from build123d import *

# Parameters (mm, degrees)
F1_DEPTH = 2.54
F2_R     = 11.6205
F3_DEPTH = 9.525
F4_SIZE  = 0.635
F5_R     = 3.175
F6_DEPTH = 2.541


with BuildPart() as f1:
    # F0 (on Top) → F1 (new body)
    with BuildSketch(Plane.XY):
        with BuildLine():
            Line((25.4, 4.7625), (8.951913, 10.724932))
            ThreePointArc((8.951913, 10.724932), (-13.97, 0), (8.951913, -10.724932))
            Line((8.951913, -10.724932), (25.4, -4.7625))
            ThreePointArc((25.4, -4.7625), (30.1625, 0), (25.4, 4.7625))
        make_face()
    extrude(amount=F1_DEPTH)

    # F2 (on face) → F3 (join)
    with BuildSketch(Plane.XY.offset(2.54)):
        with BuildLine():
            ThreePointArc((8.951913, -10.724932), (12.653441, -5.920417), (13.97, 0))
            ThreePointArc((13.97, 0), (12.653441, 5.920417), (8.951913, 10.724932))
            ThreePointArc((8.951913, 10.724932), (-13.97, 0), (8.951913, -10.724932))
        make_face()
        Circle(F2_R, mode=Mode.SUBTRACT)
    extrude(amount=F3_DEPTH)

    # F4
    f4_edges = [f1.edges().sort_by_distance(p)[0] for p in [
        (-11.6205, 0, 12.065),
    ]]
    chamfer(f4_edges, length=F4_SIZE)

    # F5 (on face) → F6 (cut, through all)
    with BuildSketch(Plane.XY.offset(2.54)):
        with Locations((25.4, 0)):
            Circle(F5_R)
    extrude(amount=-F6_DEPTH, mode=Mode.SUBTRACT)


solid = f1.part
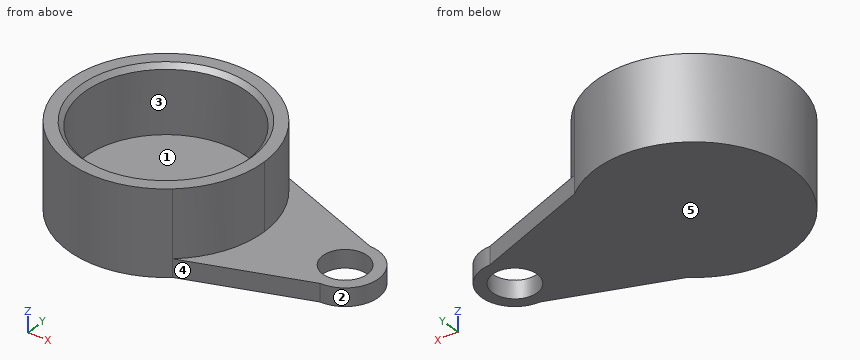
Source: CAD feature listing. Evaluate the final solid. Frame: model axes, mm. Face numbers are marked on the shaded views. A direction names the side the tool comes from. Give positions to 0.01 mm unless a question says otherwise; leave off trailing zeros. Write each loop counter-clockwise with the first axis right and the second up, starting at its lowest first coordinate (ties: lowest second). Pieces come first, ordered by that corner, then holes. Notation, with made-up numbers: M 37,34.5 L 89,34.5 A16 cw 89,58.5 Z; hole C -21,33 d4. An arc over 180 degrees is marked long. Return JSON: item names as keys, results as strings. Group by question number.
1) Material intervals for line 1 along X through (y, z) = (0.25, 9); line 2 along Y through (x, z) = (25.4, 0.6) (1 decimal); line 3 along Z through (x, y) = (1, -8.5), sorted ascending. Write a range as [from, to].
2) Cut plane C-C, the plane z = 7. Output: boundary loops of the cut face in (x, y), plus the area to 3 significant figures.
3) Pin query (flat end, axial travel): P1, Ø10.5, axis at x = 24.5, y = 3.5, coming from the +Z side; P2, Ø5, axis at y = 0.5, z = 8, coming from the +X side; P3, Ø4, axis at x = 12.5, z = 2.5, coming from the -Y side. Return the tip coordinate at first contact, or that it passes through.
4) Cut plane A-A, the plane x = 0. Output: boundary loops of the cut face in (y, z) (1 decimal), plus the area to 3 significant figures.
5) Set-up query: the marked faces 1 and 2. Return all of +Z, -Z, +X, -X, +Y, -Y with unobstructed straight access to the full face (end or side cutting, diameter ignored); none if empty.
6) Pull-direction query (Y, two-part tool) for the marked faces 3, 4 and 5; classes: pulls with the +Y half, pulls with the -Y half, needs draft (parallel to the pull), parting line crosses it, or undercut.
7) Cut plane D-D, the plane x = 15. Output: boundary loops of the cut face in (y, z), plus the area to 3 significant figures.
Recorded:
{
 "1": {"line 1": "x = [-13.97, -11.62], [11.62, 13.97]", "line 2": "y = [-4.8, -3.2], [3.2, 4.8]", "line 3": "z = [0, 2.54]"},
 "2": {"outline": "C 0,0 d27.94; hole C 0,0 d23.24", "area": "189 mm²"},
 "3": {"P1": "stops at z = 2.54", "P2": "stops at x = 13.97", "P3": "stops at y = -10.16"},
 "4": {"outline": "M -14,0 L 14,0 L 14,12.1 L 12.3,12.1 L 11.6,11.4 L 11.6,2.5 L -11.6,2.5 L -11.6,11.4 L -12.3,12.1 L -14,12.1 Z", "area": "115 mm²"},
 "5": {"face 1": "+Z", "face 2": "+Z, -Z, +X"},
 "6": {"face 3": "undercut", "face 4": "pulls with the -Y half", "face 5": "needs draft"},
 "7": {"outline": "M -8.53,0 L 8.53,0 L 8.53,2.54 L -8.53,2.54 Z", "area": "43.3 mm²"}
}
